Verification items for this drawing (mm, ordinates from the low corner). A direction names the side the tool comes from. Round coordinates to 2 decimals unless told otherwise and drop trailing zeros. Write each loop counter-clockwise with the first axis right and the second up, starting at its lowest first coordinate (ties: lowest second). Pieces come first, ordered by that corner, then holes.
Item 1: Cross-section at D-D (x = 7.75). Enter the section's corners in (y, z), then the cut area to 3 significant figures.
Item 2: Access from +Z, -Z, +X, -X, +Y, -Y to the whole of each face (thin tool, end or side, straight path). Record for the marked faces 1, 2 and 3.
Item 3: Depth check by flat-ended pin: P1, Ø2, axis at y = 107.5, z = 14.5, coming from the +X side; P2, Ø12, axis at x = 20, z = 14.5, coming from the -Y side; P3, Ø10, axis at y = 111, z = 20.5, coming from the +X side; P4, Ø12, axis at y = 45.5, z = 15, coming from the -X side. Enter the tip coordinate at first touch or a pass-through.
Item 4: Cross-section at C-C (x = 17.5). Enter the section's corners in (y, z), then the cut area to 3 significant figures.
Item 5: Cross-section at B-B (y = 12.5). Enter the section's corners in (x, z).
Item 6: Scan lines: probe 1 along Y at (x, z) = (16.25, 12.25); probe 2 along X at (y, z) = (51, 12.5); probe 3 along Y at (x, z) = (3.75, 12.5). Record each from-to range of solid material in increasing order.
Item 7: Cross-section at A-A (z = 12.5). Enter the section's corners in (x, y), then the cut area to 3 significant figures.
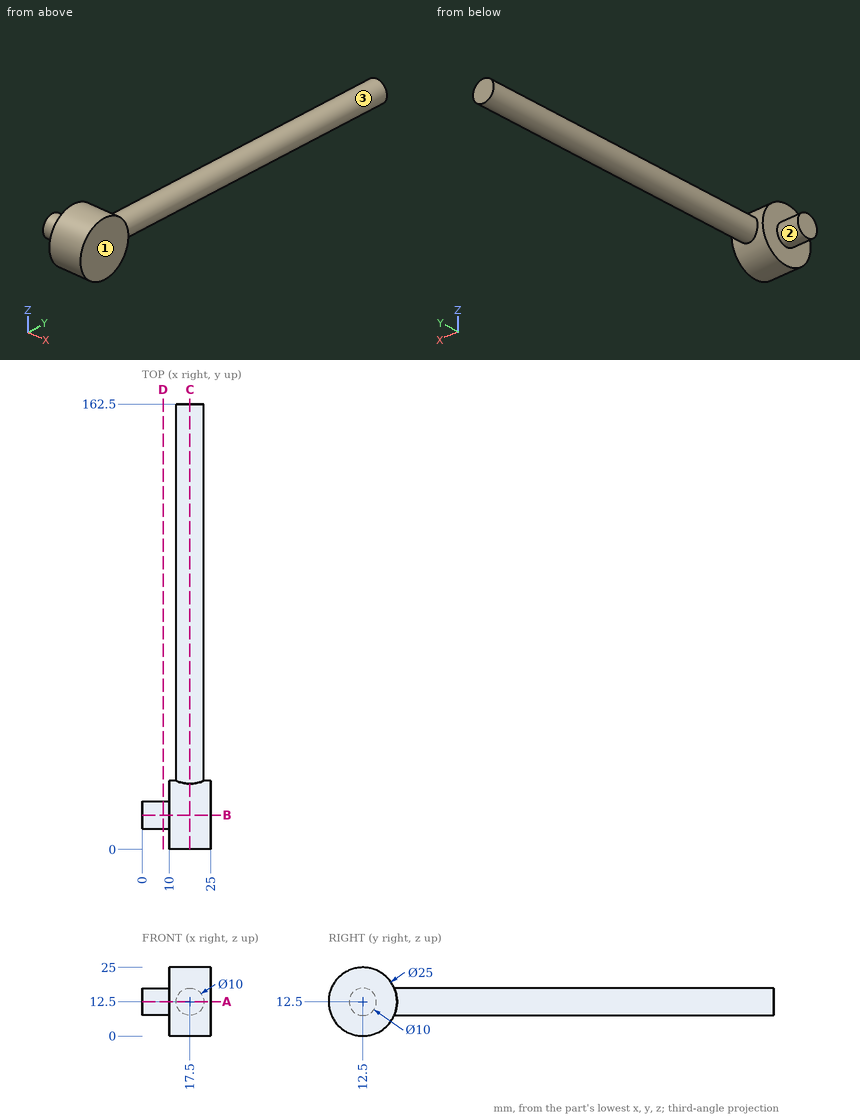
Resolved:
1. outline: circle Ø10 at (12.5, 12.5)
1. area: 78.5 mm2
2. face 1: +Z, -Z, +X, +Y, -Y
2. face 2: -X
2. face 3: +Y
3. P1: stops at x = 22.4
3. P2: stops at y = 0
3. P3: stops at x = 21.5
3. P4: stops at x = 12.5
4. outline: (23.96, 7.5) - (162.5, 7.5) - (162.5, 17.5) - (23.96, 17.5) arc R12.5 ccw (long way) to start
4. area: 1,870 mm2
5. outline: (0, 7.5) - (10, 7.5) - (10, 0) - (25, 0) - (25, 25) - (10, 25) - (10, 17.5) - (0, 17.5) - close
6. probe 1: y = 0 to 162.5
6. probe 2: x = 12.5 to 22.5
6. probe 3: y = 7.5 to 17.5
7. outline: (0, 7.5) - (10, 7.5) - (10, 0) - (25, 0) - (25, 25) - (22.5, 25) - (22.5, 162.5) - (12.5, 162.5) - (12.5, 25) - (10, 25) - (10, 17.5) - (0, 17.5) - close
7. area: 1,850 mm2
